Geometry check sheet. Reference: the model listing, model coordinates, mm. Face numbers are marked on the shaded views. A direction names the side the tool comes from. Round coordinates to 2 decimals unless told otherwise and drop trailing zeros. Order: outer loops, then holes, each group sorted by start corner. A loop starts at its lowest first (then second) coordinate and runs counter-clockwise, first axis right, second up. Notation, with made-up numbers: (45.25, -8) - (71.25, -8) arc R28 ccw to (71.25, 17) - close; hole circle Ø3 at (25, -18.5). An arc over 180 degrees is marked (long way). Write each question's results on one line, items separated by ' | '.
```python
from build123d import *

# Parameters (mm, degrees)
SKETCH1_R                = 2.73924182
BOSS_EXTRUDE1_DEPTH      = 18.034
BOSS_EXTRUDE1_DEPTH_BACK = 0.508
BOSS_EXTRUDE2_DEPTH      = 1.27


with BuildPart() as part:
    # Sketch1 → Boss-Extrude1 (new body, two sides)
    with BuildSketch(Plane.XY) as boss_extrude1_sk:
        Circle(SKETCH1_R)
    extrude(amount=BOSS_EXTRUDE1_DEPTH)
    extrude(boss_extrude1_sk.sketch, amount=-BOSS_EXTRUDE1_DEPTH_BACK)

    # Sketch2 → Boss-Extrude2 (add)
    with BuildSketch(Plane(origin=(0, 0, -0.508), x_dir=(-1, 0, 0), z_dir=(0, 0, -1))):
        Polygon((2.647524392, 3.275316604), (-1.512745189, 3.930481683), (-4.160269581, 0.655165078), (-2.647524392, -3.275316604), (1.512745189, -3.930481683), (4.160269581, -0.655165078), align=None)
    extrude(amount=BOSS_EXTRUDE2_DEPTH)


solid = part.part
```
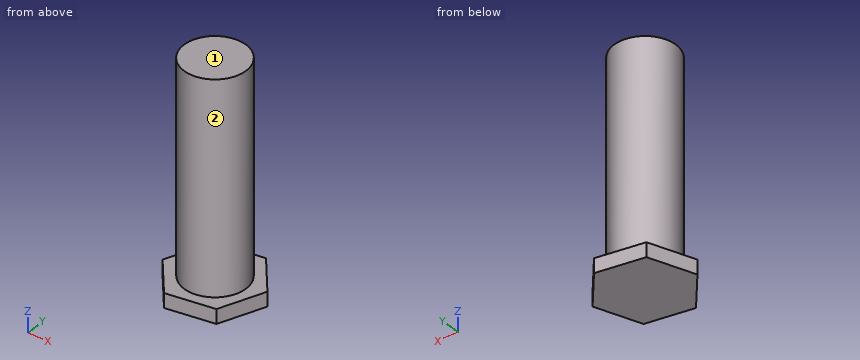
(1) Section check A-A (y = 0.25). Record the cut outline in (x, z).
Answers follow:
outline: (-3.81, -1.78) - (4, -1.78) - (4, -0.51) - (2.73, -0.51) - (2.73, 18.03) - (-2.73, 18.03) - (-2.73, -0.51) - (-3.81, -0.51) - close
(2) Access from +Z, -Z, +X, -X, +Y, -Y to the whole of each face (thin tool, end or side, straight path). Record for the marked faces 1 and 2.
Answers follow:
face 1: +Z, +X, -X, +Y, -Y | face 2: +Z
(3) Depth check by flat-ended pin: pin 1 Ø1 at (y, z) = (-2, 14.5) entering from +X; pin 2 Ø3 at (x, z) = (-2.5, 5.5) entering from -Y; pin 3 Ø1.5 at (y, z) = (2, 12.5) entering from +X. Enter the tip coordinate at first touch or a pass-through.
Answers follow:
pin 1: x = 2.29 | pin 2: y = -2.55 | pin 3: x = 2.44
(4) Material ranges on line 1 (Z direction, x = -3.5, y = 0.5); line 2 (Y direction, x = 1.5, z = 10.75); line 3 (Y direction, x = 2, z = 0.75), recorded low to high.
Answers follow:
line 1: -1.78 to -0.51 | line 2: -2.29 to 2.29 | line 3: -1.87 to 1.87
(5) Section check B-B (z = 10). Record the cut outline in (x, y).
Answers follow:
outline: circle Ø5.48 at (0, 0)
(6) Section check D-D (x = 3.5). Record the cut outline in (y, z), then the cut area to 3 significant figures.
Answers follow:
outline: (-1.06, -1.78) - (1.47, -1.78) - (1.47, -0.51) - (-1.06, -0.51) - close | area: 3.22 mm²
(7) Section check C-C (x = 0.5). Record the cut outline in (y, z).
Answers follow:
outline: (-3.61, -1.78) - (3.77, -1.78) - (3.77, -0.51) - (2.69, -0.51) - (2.69, 18.03) - (-2.69, 18.03) - (-2.69, -0.51) - (-3.61, -0.51) - close
